```python
from build123d import *

# Parameters (mm, degrees)
SKETCH1_W           = 1420
SKETCH1_H           = 19
BOSS_EXTRUDE1_DEPTH = 23.5
SKETCH2_W           = 1420
SKETCH2_H           = 16
CUT_EXTRUDE1_DEPTH  = 2.5
LPATTERN1_COUNT     = 24
LPATTERN1_PITCH     = 60
LPATTERN2_COUNT     = 24
LPATTERN2_PITCH     = 60


with BuildPart() as part:
    # Sketch1 → Boss-Extrude1 (new body)
    with BuildSketch(Plane(origin=(0, 0, 0), x_dir=(0, 0, -1), z_dir=(1, 0, 0))):
        with Locations((710, 9.5)):
            Rectangle(SKETCH1_W, SKETCH1_H)
    extrude(amount=BOSS_EXTRUDE1_DEPTH)

    # Sketch2 → Cut-Extrude1 (cut)
    with BuildSketch(Plane.ZY.offset(-23.5)):
        with Locations((-710, 11)):
            Rectangle(SKETCH2_W, SKETCH2_H)
    extrude(amount=CUT_EXTRUDE1_DEPTH, mode=Mode.SUBTRACT)

    # Sketch3 → M4x0.7 Tapped Hole1 (revolve, cut)
    with BuildSketch(Plane(origin=(0, 10.5, -28), x_dir=(0, 0, 1), z_dir=(0, 1, 0))):
        Polygon((0, 0), (0, 11.591420021), (1.65, 10.6), (1.65, 0), align=None)
    m4x0_7_tapped_hole1 = revolve(axis=Axis((-6.35, 10.5, -28), (1, 0, 0)), mode=Mode.SUBTRACT)

    # LPattern1: M4x0.7 Tapped Hole1 ×24
    with Locations(*[(0, 0, -i * LPATTERN1_PITCH) for i in range(1, LPATTERN1_COUNT)]):
        add(m4x0_7_tapped_hole1, mode=Mode.SUBTRACT)

    # Sketch5 → M3x0.5 Tapped Hole1 (revolve, cut)
    with BuildSketch(Plane(origin=(21, 10.5, -20), x_dir=(0, 0, -1), z_dir=(0, 1, 0))):
        Polygon((0, 0), (0, 10.751075774), (1.25, 10), (1.25, 0), align=None)
    m3x0_5_tapped_hole1 = revolve(axis=Axis((27.35, 10.5, -20), (-1, 0, 0)), mode=Mode.SUBTRACT)

    # LPattern2: M3x0.5 Tapped Hole1 ×24
    with Locations(*[(0, 0, -i * LPATTERN2_PITCH) for i in range(1, LPATTERN2_COUNT)]):
        add(m3x0_5_tapped_hole1, mode=Mode.SUBTRACT)


solid = part.part
```
Here's how the part is built. I have some questions about the finished solid (model axes, mm). Coordinates: 2 decimals unless noted, no trailing zeros. Order: outer loops, then holes, each group sorted by start corner. A loop starts at its lowest first (then second) coordinate and runs counter-clockwise, first axis right, second up. Notation, with made-up numbers: M 43.25,42 L 94.25,42 A11 cw 94.25,55 Z; hole C 85.5,25 d2. An arc over 180 degrees is marked long. Answer as a JSON object with one key per item and string values. Group by question number.
(1) I need wall thicknesses on probe 1 along Y at (x, z) = (4.25, -748); probe 2 along Y at (x, z) = (13.75, -500); probe 3 along X at (y, z) = (18.25, -749.5). Which ranges of each line are inside material? Lowest first, please.
(2) Suppose I cut it at A-A, the plane z = -225. Please give me the cut outline in (x, y), then the cut area to 4 significant figures.
(3) For pin 1 (5 mm diameter, centred on y = 13, z = -1055.5, fed in from +X); pin 2 (2 mm diameter, centred on y = 10.5, z = -980, fed in from +X); pin 3 (2 mm diameter, centred on y = 10.5, z = -1228, fed in from -X), each with a flat end and sliding along its axis, tell me the tip position at first contact or that it passes through.
Values found:
{
 "1": {"probe 1": "y = 0 to 8.85, 12.15 to 19", "probe 2": "y = 0 to 9.25, 11.75 to 19", "probe 3": "x = 0 to 21"},
 "2": {"outline": "M 0,0 L 23.5,0 L 23.5,3 L 21,3 L 21,19 L 0,19 Z", "area": "406.5 mm^2"},
 "3": {"pin 1": "stops at x = 21", "pin 2": "stops at x = 10.85", "pin 3": "stops at x = 10.99"}
}
